from build123d import *

# Parameters (mm, degrees)
ESBO_O1_R                = 154
RESSALTO_EXTRUS_O1_DEPTH = 16.4
ESBO_O2_R                = 145.6
CORTE_EXTRUS_O1_DEPTH    = 5.4
ESBO_O3_R                = 136.5
CORTE_EXTRUS_O2_DEPTH    = 5.72
ESBO_O4_R                = 152.8
CORTE_EXTRUS_O5_DEPTH    = 4.08


with BuildPart() as part:
    # Esboço1 → Ressalto-extrusão1 (new body)
    with BuildSketch(Plane(origin=(0, 0, 0), x_dir=(1, 0, 0), z_dir=(0, 1, 0))):
        Circle(ESBO_O1_R)
    extrude(amount=RESSALTO_EXTRUS_O1_DEPTH)

    # Esboço2 → Corte-extrusão1 (cut)
    with BuildSketch(Plane(origin=(0, 16.4, 0), x_dir=(1, 0, 0), z_dir=(0, 1, 0))):
        Circle(ESBO_O2_R)
    extrude(amount=-CORTE_EXTRUS_O1_DEPTH, mode=Mode.SUBTRACT)

    # Esboço3 → Corte-extrusão2 (cut)
    with BuildSketch(Plane(origin=(0, 11, 0), x_dir=(1, 0, 0), z_dir=(0, 1, 0))):
        Circle(ESBO_O3_R)
    extrude(amount=-CORTE_EXTRUS_O2_DEPTH, mode=Mode.SUBTRACT)

    # Esboço4 → Corte-extrusão5 (cut)
    with BuildSketch(Plane.XZ):
        Circle(ESBO_O4_R)
    extrude(amount=-CORTE_EXTRUS_O5_DEPTH, mode=Mode.SUBTRACT)


solid = part.part
Can you work these out from the model? Positions are in its coordinate system, mm. A direction names the side the tool comes from. Coordinates: 2 decimals unless noted, no trailing zeros. Order: outer loops, then holes, each group sorted by start corner. A loop starts at its lowest first (then second) coordinate and runs counter-clockwise, first axis right, second up. Notation, with made-up numbers: (-4.5, 25) -> (38.5, 25) arc R37 ccw to (38.5, 62) -> close; hole circle Ø11 at (1, -17). An arc over 180 degrees is marked (long way). Use one line per item in the form item = value.
Q1. Imagine slicing it at A-A, the plane x = 0. List the corners of the cut face in (y, z) for me.
From the geometry:
outline = (0, -154) -> (16.4, -154) -> (16.4, -145.6) -> (11, -145.6) -> (11, -136.5) -> (5.28, -136.5) -> (5.28, 136.5) -> (11, 136.5) -> (11, 145.6) -> (16.4, 145.6) -> (16.4, 154) -> (0, 154) -> (0, 152.8) -> (4.08, 152.8) -> (4.08, -152.8) -> (0, -152.8) -> close
Q2. We'd pull the mould along Z, two halves only. Please class faces 3 (the face through (-2, 5.28, -2)), 4 (the face through (-92, 16.4, 113.4)), 5 (the face through (-122.209, 8.085, 93.707)): released by +Z, released by -Z, zero draft, split by the parting line, or undercut.
From the geometry:
face_3 = undercut
face_4 = zero draft
face_5 = split by the parting line
Q3. I need wall thicknesses on L1, parallel to Z at x = 0, y = 7.35; L2, parallel to Z at x = 0, y = 1.7. Which ranges of each line are inside material? Lowest first, please.
From the geometry:
L1 = -154 to -136.5, 136.5 to 154
L2 = -154 to -152.8, 152.8 to 154
Q4. Will these pins go through, and if not, where does the flat tip stop? P1, Ø6, axis at x = 20, z = -34.5, coming from the -Y side; P2, Ø4, axis at x = -64.5, y = 6, coming from the -Z side; P3, Ø8, axis at x = -41, z = -118.5, coming from the +Y side.
From the geometry:
P1 = 4.08
P2 = -140.75
P3 = 5.28
Q5. Imagine slicing it at B-B, the plane z = -91. List the corners of the cut face in (x, y) for me.
From the geometry:
outline = (-124.24, 0) -> (-122.75, 0) -> (-122.75, 4.08) -> (122.75, 4.08) -> (122.75, 0) -> (124.24, 0) -> (124.24, 16.4) -> (113.66, 16.4) -> (113.66, 11) -> (101.74, 11) -> (101.74, 5.28) -> (-101.74, 5.28) -> (-101.74, 11) -> (-113.66, 11) -> (-113.66, 16.4) -> (-124.24, 16.4) -> close
Q6. Which directions (+Z, -Z, +X, -X, +Y, -Y) give clear straight access to the entire face, cutting with the end or side of a thin tool? Please do faces 1 (the face through (-31.56, 13.74, 142.14)), 2 (the face through (-121.257, 2.011, -92.976)).
From the geometry:
face_1 = +Y
face_2 = -Y
